```python
from build123d import *

# Parameters (mm, degrees)
SKETCH_1_W          = 126
SKETCH_1_H          = 41.5
EXTRUDE_1_DEPTH     = 1
SKETCH_2_R          = 1.6
CUT_EXTRUDE_1_DEPTH = 67.336735675
CUT_EXTRUDE_2_DEPTH = 67.336735675


with BuildPart() as part:
    # 草图1 → 凸台-拉伸1 (new body)
    with BuildSketch(Plane.XY):
        Rectangle(SKETCH_1_W, SKETCH_1_H)
    extrude(amount=EXTRUDE_1_DEPTH)

    # 草图2 → 切除-拉伸1 (cut, through all)
    with BuildSketch(Plane.XY.offset(1)):
        with Locations((-58, 15.75)):
            Circle(SKETCH_2_R)
        with Locations(Location((-58, -15.75, 0), (0, 0, 180))):
            Circle(SKETCH_2_R)
        with Locations((58, -15.75)):
            Circle(SKETCH_2_R)
        with Locations(Location((58, 15.75, 0), (0, 0, 180))):
            Circle(SKETCH_2_R)
    extrude(amount=-CUT_EXTRUDE_1_DEPTH, mode=Mode.SUBTRACT)

    # 草图3 → 切除-拉伸2 (cut, through all)
    with BuildSketch(Plane.XY.offset(1)):
        Polygon((-21.292219163, -20.75), (-18, -17.75), (18, -17.75), (21.292219163, -20.75), align=None)
    extrude(amount=-CUT_EXTRUDE_2_DEPTH, mode=Mode.SUBTRACT)


solid = part.part
```
Model file for the job. Use its own axes, mm. A direction names the side the tool comes from. Coordinates: 2 decimals unless noted, no trailing zeros. Order: outer loops, then holes, each group sorted by start corner. A loop starts at its lowest first (then second) coordinate and runs counter-clockwise, first axis right, second up. Notation, with made-up numbers: M 52,-39.75 L 109,-39.75 A30 ccw 109,-3.75 Z; hole C 43,-25 d9. An arc over 180 degrees is marked long. Answer as CSV lines item,"result".
(1) Band-saw the part on C-C, the plane y = 15.75. List the corners of the cut face in (x, z).
Geometry says:
outline,"M -63,0 L -59.6,0 L -59.6,1 L -63,1 Z; M -56.4,0 L 56.4,0 L 56.4,1 L -56.4,1 Z; M 59.6,0 L 63,0 L 63,1 L 59.6,1 Z"
(2) Band-saw the part on D-D, the plane x = -14. List the corners of the cut face in (y, z).
Geometry says:
outline,"M -17.75,0 L 20.75,0 L 20.75,1 L -17.75,1 Z"
(3) Band-saw the part on A-A, the plane x = 58. List the corners of the cut face in (y, z).
Geometry says:
outline,"M -20.75,0 L -17.35,0 L -17.35,1 L -20.75,1 Z; M -14.15,0 L 14.15,0 L 14.15,1 L -14.15,1 Z; M 17.35,0 L 20.75,0 L 20.75,1 L 17.35,1 Z"
(4) Wall check: line 1 along Y through (x, z) = (58, 0.3); line 2 along X through (y, z) = (-16, 0.25); line 3 along Y through (x, z) = (-3, 0.25). Give the ranges that are in metal, low to high.
Geometry says:
line 1,"y = -20.75 to -17.35, -14.15 to 14.15, 17.35 to 20.75"
line 2,"x = -63 to -59.58, -56.42 to 56.42, 59.58 to 63"
line 3,"y = -17.75 to 20.75"
(5) 3-axis set-ups, long thin cutter, end or side, ignore diameter. For faces 1 (the flat face through (-19.7, -19.3, 0.5)), 2 (the cylindrical face through (56.474, 15.269, 0.507)): which of +Z, -Z, +X, -X, +Y, -Y reach the whole face in a straight line?
Geometry says:
face 1,"+Z, -Z, -Y"
face 2,"+Z, -Z"
(6) Band-saw the part on B-B, the plane z = 0.45. List the corners of the cut face in (x, y).
Geometry says:
outline,"M -63,-20.75 L -21.29,-20.75 L -18,-17.75 L 18,-17.75 L 21.29,-20.75 L 63,-20.75 L 63,20.75 L -63,20.75 Z; hole C -58,-15.75 d3.2; hole C -58,15.75 d3.2; hole C 58,-15.75 d3.2; hole C 58,15.75 d3.2"
(7) Pull direction Y, two halves, no side cores. Call faces 3 (the flat face through (-1, 0, 0)), 4 (the cylindrical face through (-56.474, 16.231, 0.507)), 5 (the flat face through (19.623, -19.229, 0.507)): +Y half, -Y half, draft (parallel to the pull), parting line (faces both ways), or undercut.
Geometry says:
face 3,"draft"
face 4,"undercut"
face 5,"-Y half"
